For this review, take the finished solid that the model builds, in its own axes (mm). A direction names the side the tool comes from. Round coordinates to 2 decimals unless told otherwise and drop trailing zeros. Loops run counter-clockwise (first coordinate to the right, second up) from the corner with the lowest first, then second, coordinate; pieces in that order, holes last. Notation, with made-up numbers: (-0.5, 28.5) -> (11.5, 28.5) arc R8 cw to (11.5, 40.5) -> close; hole circle Ø7 at (85.5, 33.25). An arc over 180 degrees is marked (long way). One line per question, with ' | ' between items. Start each with the question number.
1. For faces 1 (the face through (-5.99, 45.61, 76.05)), 2 (the face through (-17, -41, 0)), list the 3-axis set-ups (+Z, -Z, +X, -X, +Y, -Y) from which the entire face can be reached by the end or side of a thin tool; tool diameter is ignored.
2. Wall thickness on line 1 along Y through (x, z) = (0, 78.5); line 2 along X through (y, z) = (-23, 53.5); line 3 along Y through (x, z) = (31, 142): over which ranges is each line inside the solid? List them lowest first.
3. Consider section B-B (z = 169.5). Write out the cut boundary in (x, y), and give its area (3 significant figures).
4. Consider section A-A (z = 78). Write out the cut boundary in (x, y), and give its area (3 significant figures).
5. For pin 1 Ø1 at (x, z) = (-47, 36.5) entering from +Y; pin 2 Ø4 at (y, z) = (12, 24.5) entering from -X; pin 3 Ø4 at (x, z) = (23.5, 113) entering from +Y; pin 4 Ø3 at (x, z) = (-15.5, 61.5) entering from +Y, all flat-tipped, find the tip position at first contact; note any pin that passes through.
```python
from build123d import *

# Parameters (mm, degrees)
F2_T = -2
F3_R = 8


with BuildPart() as f1:
    # F0 (on Front) → F1 (revolve)
    with BuildSketch(Plane.XZ):
        with BuildLine():
            Line((0, 180), (0, 0))
            Line((0, 0), (46, 0))
            Line((46, 0), (46, 150))
            ThreePointArc((46, 150), (49.9589803375, 166.7705098312), (61, 180))
            Line((61, 180), (0, 180))
        make_face()
    revolve(axis=Axis((0, 0, 90), (0, 0, 1)))

    # F2
    f2_openings = [f1.faces().sort_by_distance(p)[0] for p in [
        (0, 0, 180),
        (0, 0, 0),
    ]]
    offset(amount=F2_T, openings=f2_openings)

    # F3
    f3_edges = [f1.edges().sort_by_distance(p)[0] for p in [
        (-57.80467, 0, 180),
    ]]
    fillet(f3_edges, radius=F3_R)


solid = f1.part
```
Answer block:
1) face 1: -Z | face 2: -Z, +X, -X, +Y, -Y
2) line 1: y = -46 to -44, 44 to 46 | line 2: x = -39.84 to -37.51, 37.51 to 39.84 | line 3: y = -33.99 to -31.22, 31.22 to 33.99
3) outline: circle Ø102.94 at (0, 0); hole circle Ø98.3 at (0, 0) | area: 733 mm2
4) outline: circle Ø92 at (0, 0); hole circle Ø88 at (0, 0) | area: 565 mm2
5) pin 1: passes through | pin 2: stops at x = -44.9 | pin 3: stops at y = 40.67 | pin 4: stops at y = 43.82
